Geometry check sheet. Reference: the model listing, model coordinates, mm. A direction names the side the tool comes from. Round coordinates to 2 decimals unless told otherwise and drop trailing zeros. Write each loop counter-clockwise with the first axis right and the second up, starting at its lowest first coordinate (ties: lowest second). Pieces come first, ordered by that corner, then holes.
Item 1: Access from +Z, -Z, +X, -X, +Y, -Y to the whole of each face (thin tool, end or side, straight path). Record for faces 4 (the face through (48.83, 4.16, -9.86)), 5 (the face through (-11.2, 47.8, -9.9)), 6 (the face through (25.444, -42.009, -9.86)).
Item 2: Draft check along X on faces 1 (the face through (-11, -11, -20)), 2 (the face through (-4.16, 48.83, -9.86)), 3 (the face through (42.009, 25.444, -9.86)). Enter one of: pulls with the +X half, pulls with the -X half, needs draft (parallel to the pull), parting line crosses it, or undercut.
Item 3: Cross-section at D-D (x = 16.5). Enter the section's corners in (y, z), then the cut area to 3 significant figures.
Item 4: Cross-section at B-B (y = 0). Enter the section's corners in (x, z), then the cut area to 3 significant figures.
Item 5: Depth check by flat-ended pin: P1, Ø12, axis at x = -30, z = -14, coming from the +Y side; P2, Ø24, axis at x = 0, y = 0, coming from the +Z side; P3, Ø6, axis at x = 9.5, z = -10, coming from the -Y side; P4, Ø1.1, axis at y = 14.5, z = -8, coming from the -X side. Enter the tip coordinate at first touch or a pass-through.
Item 6: Cross-section at A-A (x = 0). Enter the section's corners in (y, z), then the cut area to 3 significant figures.
Item 7: Cross-section at C-C (y = -38.5). Enter the section's corners in (x, z), then the cut area to 3 significant figures.
Item 8: Scan lines: probe 1 along Y at (x, z) = (0, -13.75); probe 2 along X at (y, z) = (0, -9.5); probe 3 along X at (y, z) = (42.5, -18.5). Record each from-to range of solid material in increasing order.
from build123d import *

# Parameters (mm, degrees)
BOSS_EXTRUDE1_DEPTH = 20


with BuildPart() as part:
    # Sketch1 → Boss-Extrude1 (new body)
    with BuildSketch(Plane.XY):
        with BuildLine():
            Line((-1.360697771, 53.5), (1.360697771, 53.5))
            ThreePointArc((1.360697771, 53.5), (1.899334334, 53.342538221), (2.268341553, 52.919741307))
            Line((2.268341553, 52.919741307), (6, 44.850445929))
            ThreePointArc((6, 44.850445929), (7.078659543, 44.692897412), (8.153210899, 44.509410825))
            Line((8.153210899, 44.509410825), (14.195778386, 51.030620899))
            ThreePointArc((14.195778386, 51.030620899), (14.677376539, 51.318695158), (15.238308717, 51.302002357))
            Line((15.238308717, 51.302002357), (17.826509681, 50.461044886))
            ThreePointArc((17.826509681, 50.461044886), (18.290125128, 50.144841983), (18.510420417, 49.628708722))
            Line((18.510420417, 49.628708722), (19.565889095, 40.801206893))
            ThreePointArc((19.565889095, 40.801206893), (20.543070113, 40.31804522), (21.508328709, 39.811484475))
            Line((21.508328709, 39.811484475), (29.27031663, 44.146267767))
            ThreePointArc((29.27031663, 44.146267767), (29.817363532, 44.271420654), (30.345683377, 44.082207282))
            Line((30.345683377, 44.082207282), (32.547338618, 42.482611117))
            ThreePointArc((32.547338618, 42.482611117), (32.89055104, 42.038619233), (32.940570361, 41.479672343))
            Line((32.940570361, 41.479672343), (31.216532642, 32.758061448))
            ThreePointArc((31.216532642, 32.758061448), (31.996581849, 31.996581849), (32.758061448, 31.216532642))
            Line((32.758061448, 31.216532642), (41.479672343, 32.940570361))
            ThreePointArc((41.479672343, 32.940570361), (42.038619233, 32.89055104), (42.482611117, 32.547338618))
            Line((42.482611117, 32.547338618), (44.082207282, 30.345683377))
            ThreePointArc((44.082207282, 30.345683377), (44.271420654, 29.817363532), (44.146267767, 29.27031663))
            Line((44.146267767, 29.27031663), (39.811484475, 21.508328709))
            ThreePointArc((39.811484475, 21.508328709), (40.31804522, 20.543070113), (40.801206893, 19.565889095))
            Line((40.801206893, 19.565889095), (49.628708722, 18.510420417))
            ThreePointArc((49.628708722, 18.510420417), (50.144841983, 18.290125128), (50.461044886, 17.826509681))
            Line((50.461044886, 17.826509681), (51.302002357, 15.238308717))
            ThreePointArc((51.302002357, 15.238308717), (51.318695158, 14.677376539), (51.030620899, 14.195778386))
            Line((51.030620899, 14.195778386), (44.509410825, 8.153210899))
            ThreePointArc((44.509410825, 8.153210899), (44.692897412, 7.078659543), (44.850445929, 6))
            Line((44.850445929, 6), (52.919741307, 2.268341553))
            ThreePointArc((52.919741307, 2.268341553), (53.342538221, 1.899334334), (53.5, 1.360697771))
            Line((53.5, 1.360697771), (53.5, -1.360697771))
            ThreePointArc((53.5, -1.360697771), (53.342538221, -1.899334334), (52.919741307, -2.268341553))
            Line((52.919741307, -2.268341553), (44.850445929, -6))
            ThreePointArc((44.850445929, -6), (44.692897412, -7.078659543), (44.509410825, -8.153210899))
            Line((44.509410825, -8.153210899), (51.030620899, -14.195778386))
            ThreePointArc((51.030620899, -14.195778386), (51.318695158, -14.677376539), (51.302002357, -15.238308717))
            Line((51.302002357, -15.238308717), (50.461044886, -17.826509681))
            ThreePointArc((50.461044886, -17.826509681), (50.144841983, -18.290125128), (49.628708722, -18.510420417))
            Line((49.628708722, -18.510420417), (40.801206893, -19.565889095))
            ThreePointArc((40.801206893, -19.565889095), (40.31804522, -20.543070113), (39.811484475, -21.508328709))
            Line((39.811484475, -21.508328709), (44.146267767, -29.27031663))
            ThreePointArc((44.146267767, -29.27031663), (44.271420654, -29.817363532), (44.082207282, -30.345683377))
            Line((44.082207282, -30.345683377), (42.482611117, -32.547338618))
            ThreePointArc((42.482611117, -32.547338618), (42.038619233, -32.89055104), (41.479672343, -32.940570361))
            Line((41.479672343, -32.940570361), (32.758061448, -31.216532642))
            ThreePointArc((32.758061448, -31.216532642), (31.996581849, -31.996581849), (31.216532642, -32.758061448))
            Line((31.216532642, -32.758061448), (32.940570361, -41.479672343))
            ThreePointArc((32.940570361, -41.479672343), (32.89055104, -42.038619233), (32.547338618, -42.482611117))
            Line((32.547338618, -42.482611117), (30.345683377, -44.082207282))
            ThreePointArc((30.345683377, -44.082207282), (29.817363532, -44.271420654), (29.27031663, -44.146267767))
            Line((29.27031663, -44.146267767), (21.508328709, -39.811484475))
            ThreePointArc((21.508328709, -39.811484475), (20.543070113, -40.31804522), (19.565889095, -40.801206893))
            Line((19.565889095, -40.801206893), (18.510420417, -49.628708722))
            ThreePointArc((18.510420417, -49.628708722), (18.290125128, -50.144841983), (17.826509681, -50.461044886))
            Line((17.826509681, -50.461044886), (15.238308717, -51.302002357))
            ThreePointArc((15.238308717, -51.302002357), (14.677376539, -51.318695158), (14.195778386, -51.030620899))
            Line((14.195778386, -51.030620899), (8.153210899, -44.509410825))
            ThreePointArc((8.153210899, -44.509410825), (7.078659543, -44.692897412), (6, -44.850445929))
            Line((6, -44.850445929), (2.268341553, -52.919741307))
            ThreePointArc((2.268341553, -52.919741307), (1.899334334, -53.342538221), (1.360697771, -53.5))
            Line((1.360697771, -53.5), (-1.360697771, -53.5))
            ThreePointArc((-1.360697771, -53.5), (-1.899334334, -53.342538221), (-2.268341553, -52.919741307))
            Line((-2.268341553, -52.919741307), (-6, -44.850445929))
            ThreePointArc((-6, -44.850445929), (-7.078659543, -44.692897412), (-8.153210899, -44.509410825))
            Line((-8.153210899, -44.509410825), (-14.195778386, -51.030620899))
            ThreePointArc((-14.195778386, -51.030620899), (-14.677376539, -51.318695158), (-15.238308717, -51.302002357))
            Line((-15.238308717, -51.302002357), (-17.826509681, -50.461044886))
            ThreePointArc((-17.826509681, -50.461044886), (-18.290125128, -50.144841983), (-18.510420417, -49.628708722))
            Line((-18.510420417, -49.628708722), (-19.565889095, -40.801206893))
            ThreePointArc((-19.565889095, -40.801206893), (-20.543070113, -40.31804522), (-21.508328709, -39.811484475))
            Line((-21.508328709, -39.811484475), (-29.27031663, -44.146267767))
            ThreePointArc((-29.27031663, -44.146267767), (-29.817363532, -44.271420654), (-30.345683377, -44.082207282))
            Line((-30.345683377, -44.082207282), (-32.547338618, -42.482611117))
            ThreePointArc((-32.547338618, -42.482611117), (-32.89055104, -42.038619233), (-32.940570361, -41.479672343))
            Line((-32.940570361, -41.479672343), (-31.216532642, -32.758061448))
            ThreePointArc((-31.216532642, -32.758061448), (-31.996581849, -31.996581849), (-32.758061448, -31.216532642))
            Line((-32.758061448, -31.216532642), (-41.479672343, -32.940570361))
            ThreePointArc((-41.479672343, -32.940570361), (-42.038619233, -32.89055104), (-42.482611117, -32.547338618))
            Line((-42.482611117, -32.547338618), (-44.082207282, -30.345683377))
            ThreePointArc((-44.082207282, -30.345683377), (-44.271420654, -29.817363532), (-44.146267767, -29.27031663))
            Line((-44.146267767, -29.27031663), (-39.811484475, -21.508328709))
            ThreePointArc((-39.811484475, -21.508328709), (-40.31804522, -20.543070113), (-40.801206893, -19.565889095))
            Line((-40.801206893, -19.565889095), (-49.628708722, -18.510420417))
            ThreePointArc((-49.628708722, -18.510420417), (-50.144841983, -18.290125128), (-50.461044886, -17.826509681))
            Line((-50.461044886, -17.826509681), (-51.302002357, -15.238308717))
            ThreePointArc((-51.302002357, -15.238308717), (-51.318695158, -14.677376539), (-51.030620899, -14.195778386))
            Line((-51.030620899, -14.195778386), (-44.509410825, -8.153210899))
            ThreePointArc((-44.509410825, -8.153210899), (-44.692897412, -7.078659543), (-44.850445929, -6))
            Line((-44.850445929, -6), (-52.919741307, -2.268341553))
            ThreePointArc((-52.919741307, -2.268341553), (-53.342538221, -1.899334334), (-53.5, -1.360697771))
            Line((-53.5, -1.360697771), (-53.5, 1.360697771))
            ThreePointArc((-53.5, 1.360697771), (-53.342538221, 1.899334334), (-52.919741307, 2.268341553))
            Line((-52.919741307, 2.268341553), (-44.850445929, 6))
            ThreePointArc((-44.850445929, 6), (-44.692897412, 7.078659543), (-44.509410825, 8.153210899))
            Line((-44.509410825, 8.153210899), (-51.030620899, 14.195778386))
            ThreePointArc((-51.030620899, 14.195778386), (-51.318695158, 14.677376539), (-51.302002357, 15.238308717))
            Line((-51.302002357, 15.238308717), (-50.461044886, 17.826509681))
            ThreePointArc((-50.461044886, 17.826509681), (-50.144841983, 18.290125128), (-49.628708722, 18.510420417))
            Line((-49.628708722, 18.510420417), (-40.801206893, 19.565889095))
            ThreePointArc((-40.801206893, 19.565889095), (-40.31804522, 20.543070113), (-39.811484475, 21.508328709))
            Line((-39.811484475, 21.508328709), (-44.146267767, 29.27031663))
            ThreePointArc((-44.146267767, 29.27031663), (-44.271420654, 29.817363532), (-44.082207282, 30.345683377))
            Line((-44.082207282, 30.345683377), (-42.482611117, 32.547338618))
            ThreePointArc((-42.482611117, 32.547338618), (-42.038619233, 32.89055104), (-41.479672343, 32.940570361))
            Line((-41.479672343, 32.940570361), (-32.758061448, 31.216532642))
            ThreePointArc((-32.758061448, 31.216532642), (-31.996581849, 31.996581849), (-31.216532642, 32.758061448))
            Line((-31.216532642, 32.758061448), (-32.940570361, 41.479672343))
            ThreePointArc((-32.940570361, 41.479672343), (-32.89055104, 42.038619233), (-32.547338618, 42.482611117))
            Line((-32.547338618, 42.482611117), (-30.345683377, 44.082207282))
            ThreePointArc((-30.345683377, 44.082207282), (-29.817363532, 44.271420654), (-29.27031663, 44.146267767))
            Line((-29.27031663, 44.146267767), (-21.508328709, 39.811484475))
            ThreePointArc((-21.508328709, 39.811484475), (-20.543070113, 40.31804522), (-19.565889095, 40.801206893))
            Line((-19.565889095, 40.801206893), (-18.510420417, 49.628708722))
            ThreePointArc((-18.510420417, 49.628708722), (-18.290125128, 50.144841983), (-17.826509681, 50.461044886))
            Line((-17.826509681, 50.461044886), (-15.238308717, 51.302002357))
            ThreePointArc((-15.238308717, 51.302002357), (-14.677376539, 51.318695158), (-14.195778386, 51.030620899))
            Line((-14.195778386, 51.030620899), (-8.153210899, 44.509410825))
            ThreePointArc((-8.153210899, 44.509410825), (-7.078659543, 44.692897412), (-6, 44.850445929))
            Line((-6, 44.850445929), (-2.268341553, 52.919741307))
            ThreePointArc((-2.268341553, 52.919741307), (-1.899334334, 53.342538221), (-1.360697771, 53.5))
        make_face()
        with BuildLine():
            Line((6, 13.747727085), (6, 15.997727085))
            Line((6, 15.997727085), (-6, 15.997727085))
            Line((-6, 15.997727085), (-6, 13.747727085))
            ThreePointArc((-6, 13.747727085), (0, -15), (6, 13.747727085))
        make_face(mode=Mode.SUBTRACT)
    extrude(amount=-BOSS_EXTRUDE1_DEPTH)


solid = part.part
Resolved:
1. face 4: +Z, -Z, +X
1. face 5: +Z, -Z, +Y
1. face 6: +Z, -Z, -Y
2. face 1: needs draft
2. face 2: undercut
2. face 3: pulls with the +X half
3. outline: (-50.89, -20) - (50.89, -20) - (50.89, 0) - (-50.89, 0) - close
3. area: 2,040 mm2
4. outline: (-53.5, -20) - (-15, -20) - (-15, 0) - (-53.5, 0) - close; (15, -20) - (53.5, -20) - (53.5, 0) - (15, 0) - close
4. area: 1,540 mm2
5. P1: stops at y = 44.27
5. P2: passes through
5. P3: stops at y = -49.2
5. P4: stops at x = -51.35
6. outline: (-53.5, -20) - (-15, -20) - (-15, 0) - (-53.5, 0) - close; (16, -20) - (53.5, -20) - (53.5, 0) - (16, 0) - close
6. area: 1,520 mm2
7. outline: (-32.35, -20) - (32.35, -20) - (32.35, 0) - (-32.35, 0) - close
7. area: 1,290 mm2
8. probe 1: y = -53.5 to -15, 16 to 53.5
8. probe 2: x = -53.5 to -15, 15 to 53.5
8. probe 3: x = -32.52 to -26.32, -19.36 to 19.36, 26.32 to 32.52
